The model under review builds one solid part; all positions refer to its coordinate system, in mm. A direction names the side the tool comes from. Give positions to 0.01 mm unless a question says otherwise; leave off trailing zeros. Write each loop counter-clockwise with the first axis right and the second up, starting at its lowest first coordinate (ties: lowest second). Pieces come first, ordered by that corner, then holes. Notation, with made-up numbers: (-36.5, 57) - (-17.5, 57) arc R13 ccw to (-17.5, 73) - close; hole circle Ø11 at (-31.5, 74.5). An arc over 180 degrees is marked (long way). Write item = value, one per line.
```python
from build123d import *

# Parameters (mm, degrees)
F1_DEPTH = 25.4
F2_R     = 5.08


with BuildPart() as f1:
    # F0 (on Top) → F1 (new body)
    with BuildSketch(Plane.XY):
        Polygon((0, 127), (-117.475, 127), (-117.475, -25.4), (-136.525, -25.4), (-136.525, -127), (0, -127), align=None)
        Polygon((117.475, 127), (0, 127), (0, -127), (136.525, -127), (136.525, -25.4), (117.475, -25.4), align=None)
    extrude(amount=F1_DEPTH)

    # F2
    f2_edges = [f1.edges().sort_by_distance(p)[0] for p in [
        (0, -127, 0),
        (-117.475, 50.8, 25.4),
        (117.475, 50.8, 0),
        (136.525, -76.2, 25.4),
        (127, -25.4, 25.4),
        (117.475, 127, 12.7),
        (136.525, -76.2, 0),
        (-136.525, -76.2, 25.4),
        (117.475, 50.8, 25.4),
        (0, -127, 25.4),
        (0, 127, 25.4),
        (136.525, -25.4, 12.7),
        (-127, -25.4, 0),
        (-127, -25.4, 25.4),
        (-136.525, -25.4, 12.7),
        (-117.475, 50.8, 0),
        (0, 127, 0),
        (-136.525, -127, 12.7),
        (136.525, -127, 12.7),
        (117.475, -25.4, 12.7),
        (-136.525, -76.2, 0),
        (-117.475, -25.4, 12.7),
        (-117.475, 127, 12.7),
        (127, -25.4, 0),
    ]]
    fillet(f2_edges, radius=F2_R)


solid = f1.part
```
1. For line 1 (X direction, y = 39, z = 14.75) (3 decimals); line 2 (X direction, y = 72, z = 21.5); line 3 (Y direction, x = -106, z = 22), list the stretches that pass through material, from the lowest coordinate up. Write a range as from..to.
Findings below:
line_1 = -117.475..117.475
line_2 = -117.34..117.34
line_3 = -126.71..126.71
2. Take a section at A-A on z = 11.5. Give the boundary of the cut face in (x, y) (3 decimals).
Findings below:
outline = (-136.525, -121.92) arc R5.08 ccw to (-131.445, -127) - (131.445, -127) arc R5.08 ccw to (136.525, -121.92) - (136.525, -30.48) arc R5.08 ccw to (131.445, -25.4) - (122.555, -25.4) arc R5.08 cw to (117.475, -20.32) - (117.475, 121.92) arc R5.08 ccw to (112.395, 127) - (-112.395, 127) arc R5.08 ccw to (-117.475, 121.92) - (-117.475, -20.32) arc R5.08 cw to (-122.555, -25.4) - (-131.445, -25.4) arc R5.08 ccw to (-136.525, -30.48) - close
3. Machinability: for faces 1 (the flat face through (-127, -25.4, 13)), 2 (the flat face through (-2, 2, 25.4)), 3 (the flat face through (127, -25.4, 13)), which of the approach directions +Z, -Z, +X, -X, +Y, -Y give a long, thin tool a straight path to every point of the face, cutting with its end or side? Answer none if there is none.
Findings below:
face_1 = +Z, -Z, -X, +Y
face_2 = +Z, +X, -X, +Y, -Y
face_3 = +Z, -Z, +X, +Y
4. Take a section at B-B on y = 95.5. Give the boundary of the cut face in (x, z) (3 decimals).
Findings below:
outline = (-117.475, 5.08) arc R5.08 ccw to (-112.395, 0) - (112.395, 0) arc R5.08 ccw to (117.475, 5.08) - (117.475, 20.32) arc R5.08 ccw to (112.395, 25.4) - (-112.395, 25.4) arc R5.08 ccw to (-117.475, 20.32) - close
5. Insertion check: P1, Ø12, axis at y = 54, z = 10.5, coming from the +X side (3 decimals); P2, Ø2.5, axis at x = 128, z = 9.5, coming from the +Y side; P3, Ø10, axis at x = -125, z = 11.5, coming from the +Y side. Each pin has a flat end and moves straight along its axis. Give the tip position at first contact, or say it passes through.
Findings below:
P1 = 117.475
P2 = -25.4
P3 = -24.71
